Build history of the part. All positions in model axes, mm. Round coordinates to 2 decimals unless told otherwise and drop trailing zeros. Write each loop counter-clockwise with the first axis right and the second up, starting at its lowest first coordinate (ties: lowest second). Pieces come first, ordered by that corner, then holes. Notation, with made-up numbers: M 34,71 L 76,71 A27 ccw 76,108 Z; hole C 25.5,-4 d1. An arc over 180 degrees is marked long. Write item = value, one per line. Start each with the question number.
Q1. Band-saw the part on D-D on y = 1.5. Write the cut outline in (x, z).
Q2. Band-saw the part on B-B on x = -30. Write the cut outline in (y, z), plus the area to 3 significant figures.
Q3. Drop flat-ended pins along their axis: P1, Ø5, axis at x = 31.5, z = 12.5, coming from the -Y side; P2, Ø13.5, axis at x = 10, z = 20, coming from the -Y side. Give the stop position or say it passes through.
Q4. Band-saw the part on A-A on y = 7. Write the cut outline in (x, z).
Q5. Band-saw the part on C-C on z = 20. Write the cut outline in (x, y), plus the area to 3 significant figures.
Q6. Pull direction Z, two halves, no side cores. Call faces 1 (the flat face through (-1, 5, 40)), 2 (the cylindrical face through (-49.044, 4.93, -39.093)), 3 (the cylindrical face through (41.986, 5.07, -19.177)): released by +Z, released by -Z, zero draft, split by the parting line, or undercut.
Q7. Probe L1, parallel to Z at x = -30, y = 8.7; L2, parallel to X at y = 8.55, z = -20; L3, parallel to Z at x = 40, y = 4.5. List the from-to ranges inside material, lowest first.
```python
from build123d import *

# Parameters (mm, degrees)
BOSS_EXTRUDE1_DEPTH                             = 10
CSK_FOR_M8_FLAT_HEAD_MACHINE_SCREW1_D           = 8.4
CSK_FOR_M8_FLAT_HEAD_MACHINE_SCREW1_CSINK_D     = 17.3
CSK_FOR_M8_FLAT_HEAD_MACHINE_SCREW1_CSINK_ANGLE = 90
M4_CLEARANCE_HOLE1_D                            = 4.3


with BuildPart() as part:
    # Sketch1 → Boss-Extrude1 (new body)
    with BuildSketch(Plane(origin=(0, 0, 0), x_dir=(1, 0, 0), z_dir=(0, 1, 0))):
        with BuildLine():
            Line((-46.82, -40), (46.82, -40))
            ThreePointArc((46.82, -40), (49.068599564, -39.068599564), (50, -36.82))
            Line((50, -36.82), (50, 36.82))
            ThreePointArc((50, 36.82), (49.068599564, 39.068599564), (46.82, 40))
            Line((46.82, 40), (-46.82, 40))
            ThreePointArc((-46.82, 40), (-49.068599564, 39.068599564), (-50, 36.82))
            Line((-50, 36.82), (-50, -36.82))
            ThreePointArc((-50, -36.82), (-49.068599564, -39.068599564), (-46.82, -40))
        make_face()
    extrude(amount=BOSS_EXTRUDE1_DEPTH)

    # CSK for M8 Flat Head Machine Screw1 (through all)
    with Locations(Plane(origin=(0, 0, 0), x_dir=(-1, 0, 0), z_dir=(0, -1, 0))):
        with Locations((-10, 20), (30, 20), (30, -20), (-10, -20)):
            CounterSinkHole(CSK_FOR_M8_FLAT_HEAD_MACHINE_SCREW1_D / 2, CSK_FOR_M8_FLAT_HEAD_MACHINE_SCREW1_CSINK_D / 2, counter_sink_angle=CSK_FOR_M8_FLAT_HEAD_MACHINE_SCREW1_CSINK_ANGLE)

    # M4 Clearance Hole1 (through all)
    with Locations(Plane(origin=(0, 0, 0), x_dir=(-1, 0, 0), z_dir=(0, -1, 0))):
        with Locations((-40, 20), (-40, -20)):
            Hole(M4_CLEARANCE_HOLE1_D / 2)


solid = part.part
```
Conclusion:
q1.outline = M -50,-36.82 A3.18 ccw -46.82,-40 L 46.82,-40 A3.18 ccw 50,-36.82 L 50,36.82 A3.18 ccw 46.82,40 L -46.82,40 A3.18 ccw -50,36.82 Z; hole C -30,-20 d14.3; hole C -30,20 d14.3; hole C 10,-20 d14.3; hole C 10,20 d14.3; hole C 40,-20 d4.3; hole C 40,20 d4.3
q2.outline = M 0,-40 L 10,-40 L 10,-24.2 L 4.45,-24.2 L 0,-28.65 Z; M 0,-11.35 L 4.45,-15.8 L 10,-15.8 L 10,15.8 L 4.45,15.8 L 0,11.35 Z; M 0,28.65 L 4.45,24.2 L 10,24.2 L 10,40 L 0,40 Z
q2.area = 592 mm^2
q3.P1 = 0
q3.P2 = 1.9
q4.outline = M -50,-36.82 A3.18 ccw -46.82,-40 L 46.82,-40 A3.18 ccw 50,-36.82 L 50,36.82 A3.18 ccw 46.82,40 L -46.82,40 A3.18 ccw -50,36.82 Z; hole C -30,-20 d8.4; hole C -30,20 d8.4; hole C 10,-20 d8.4; hole C 10,20 d8.4; hole C 40,-20 d4.3; hole C 40,20 d4.3
q5.outline = M -50,0 L -38.65,0 L -34.2,4.45 L -34.2,10 L -50,10 Z; M -25.8,4.45 L -21.35,0 L 1.35,0 L 5.8,4.45 L 5.8,10 L -25.8,10 Z; M 14.2,4.45 L 18.65,0 L 37.85,0 L 37.85,10 L 14.2,10 Z; M 42.15,0 L 50,0 L 50,10 L 42.15,10 Z
q5.area = 749 mm^2
q6.face_1 = released by +Z
q6.face_2 = released by -Z
q6.face_3 = undercut
q7.L1 = -40 to -24.2, -15.8 to 15.8, 24.2 to 40
q7.L2 = -50 to -34.2, -25.8 to 5.8, 14.2 to 37.85, 42.15 to 50
q7.L3 = -40 to -22.15, -17.85 to 17.85, 22.15 to 40
